Study the drawing (mm; zero at the part's minimum x, y, z) and answer. A direction names the side the tool comes from. Give positions to 0.01 mm unless a question says otherwise; leave off trailing zeros. Order: outer loops, then holes, each group sorted by start corner. A loop starts at its lowest first (then second) coordinate and runs counter-clockwise, first axis right, second up. Notation, with made-up numbers: (7, -32) - (44, -32) arc R22 cw to (44, -8) - close; hole circle Ø9 at (27.25, 46.25). An arc over 180 degrees is marked (long way). Put each result on its own line as item: value.
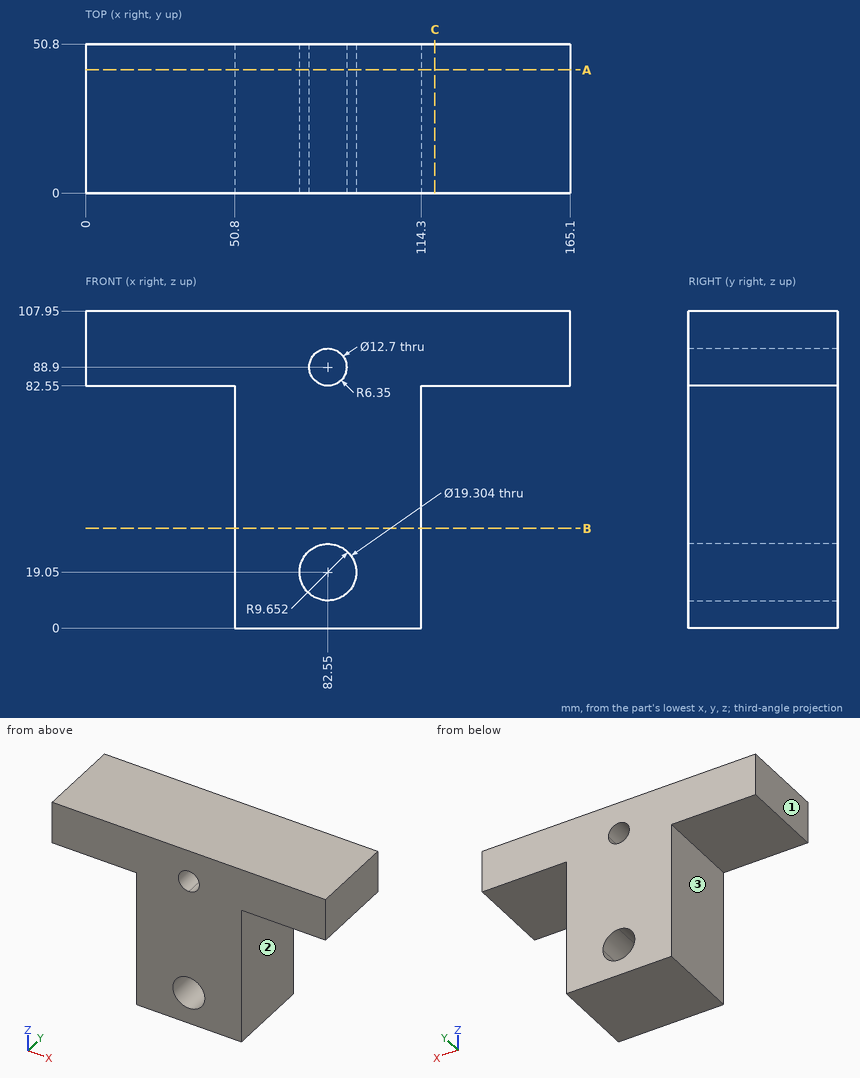
(1) Section B-B, the plane z = 34 is taken. Write down the section's boundary in (x, y), then the cut area to 3 significant figures.
Geometry check:
outline: (50.8, 0) - (114.3, 0) - (114.3, 50.8) - (50.8, 50.8) - close
area: 3,230 mm²
(2) Section A-A, the plane y = 42 is taken. Write down the section's boundary in (x, z).
Geometry check:
outline: (0, 82.55) - (50.8, 82.55) - (50.8, 0) - (114.3, 0) - (114.3, 82.55) - (165.1, 82.55) - (165.1, 107.95) - (0, 107.95) - close; hole circle Ø19.3 at (82.55, 19.05); hole circle Ø12.7 at (82.55, 88.9)
(3) Straight lines are drawn through the part: line 1 (Z direction, x = 82.55, y = 14); line 2 (X direction, y = 32, z = 19); line 3 (Z direction, x = 84, y = 40.5). For each, find the intervals that lie inside material, in ascending order.
Geometry check:
line 1: z = 0 to 9.4, 28.7 to 82.55, 95.25 to 107.95
line 2: x = 50.8 to 72.9, 92.2 to 114.3
line 3: z = 0 to 9.51, 28.59 to 82.72, 95.08 to 107.95
(4) A tool of negligible diameter and unlimited length cuts with its end or side. For the marked faces 1, 2 and 3, from which of +Z, -Z, +X, -X, +Y, -Y can it reach the whole face along a straight path? Write none if from no direction.
Geometry check:
face 1: +Z, -Z, -X, +Y, -Y
face 2: -Z, +X, +Y, -Y
face 3: -Z, -X, +Y, -Y
(5) Section C-C, the plane x = 119 is taken. Write down the section's boundary in (y, z).
Geometry check:
outline: (0, 82.55) - (50.8, 82.55) - (50.8, 107.95) - (0, 107.95) - close
(6) Given pin 1 (5 mm diameter, centred on x = 139, y = 35, fed in from -Z); pin 2 (1 mm diameter, centred on y = 30.5, z = 77.5, fed in from +X); pin 3 (1.5 mm diameter, centred on y = 10.5, z = 69, fed in from -X); pin 4 (11.5 mm diameter, centred on x = 82.55, z = 88.9, fed in from -Y), each flat-ended and moving along its own axis, determine where each tip first touches the part or whether it passes through.
Geometry check:
pin 1: stops at z = 82.55
pin 2: stops at x = 114.3
pin 3: stops at x = 50.8
pin 4: passes through
